Input: part model. Units: mm. Frame: model coordinates. A direction names the side the tool comes from. Coordinates: 2 decimals unless noted, no trailing zeros. Order: outer loops, then holes, each group sorted by start corner. A loop starts at its lowest first (then second) coordinate and runs counter-clockwise, first axis right, second up. Notation, with made-up numbers: (-25, 62.5) -> (-9, 62.5) arc R18 cw to (-9, 73.5) -> close; hole circle Ø2 at (49.5, 48). An arc over 180 degrees is marked (long way). One line per question, with ' | ' between items.
```python
from build123d import *

# Parameters (mm, degrees)
F1_DEPTH = 25.4
F3_DEPTH = 19.05


with BuildPart() as f1:
    # F0 (on Front) → F1 (new body)
    with BuildSketch(Plane.XZ):
        with BuildLine():
            Line((22.462801, 43.289483), (-25.703526, 43.289483))
            ThreePointArc((-25.703526, 43.289483), (-28.848755, 41.986686), (-30.151552, 38.841457))
            Line((-30.151552, 38.841457), (-30.151552, -42.523745))
            ThreePointArc((-30.151552, -42.523745), (-28.849641, -45.666835), (-25.706552, -46.968745))
            Line((-25.706552, -46.968745), (22.462801, -46.968745))
            ThreePointArc((22.462801, -46.968745), (25.605891, -45.666835), (26.907801, -42.523745))
            Line((26.907801, -42.523745), (26.907801, 38.844483))
            ThreePointArc((26.907801, 38.844483), (25.605891, 41.987572), (22.462801, 43.289483))
        make_face()
    extrude(amount=F1_DEPTH)

    # F2 (on face) → F3 (join)
    with BuildSketch(Plane.XZ.offset(25.4)):
        with BuildLine():
            Line((26.907801, 0), (-30.151552, 0))
            Line((-30.151552, 0), (-30.151552, -42.523745))
            ThreePointArc((-30.151552, -42.523745), (-28.849641, -45.666835), (-25.706552, -46.968745))
            Line((-25.706552, -46.968745), (22.462801, -46.968745))
            ThreePointArc((22.462801, -46.968745), (25.605891, -45.666835), (26.907801, -42.523745))
            Line((26.907801, -42.523745), (26.907801, 0))
        make_face()
    extrude(amount=F3_DEPTH)


solid = f1.part
```
1. Cut plane A-A, the plane y = -27.5. Return loops of the section in (x, z) (3 decimals), and give its area (3 significant figures).
Recorded:
outline: (-30.152, -42.524) arc R4.445 ccw to (-25.707, -46.969) -> (22.463, -46.969) arc R4.445 ccw to (26.908, -42.524) -> (26.908, 0) -> (-30.152, 0) -> close | area: 2,670 mm^2
2. Cut plane B-B, the plane x = 21.5. Return loops of the section in (y, z).
Recorded:
outline: (-44.45, -46.97) -> (0, -46.97) -> (0, 43.29) -> (-25.4, 43.29) -> (-25.4, 0) -> (-44.45, 0) -> close
3. Ray query, line 1 (Y direction, x = -21, z = 22); line 2 (Z direction, x = 13, y = -26.5); line 3 (Z direction, x = -27.5, y = -10). Return the intervals inside material, ascending. Write a range as [from, to].
Recorded:
line 1: y = [-25.4, 0] | line 2: z = [-46.97, 0] | line 3: z = [-46.59, 42.91]
4. Pin query (flat end, axial travel): pin 1 Ø5 at (x, y) = (18.5, -26) entering from +Z; pin 2 Ø9.5 at (x, y) = (6, -32) entering from +Z; pin 3 Ø21.5 at (x, z) = (10.5, 19.5) entering from -Y. Return the tip coordinate at first contact, or that it passes through.
Recorded:
pin 1: stops at z = 43.29 | pin 2: stops at z = 0 | pin 3: stops at y = -25.4
5. Cut plane C-C, the plane z = 31. Return loops of the section in (x, y), and give its area (3 significant figures).
Recorded:
outline: (-30.15, -25.4) -> (26.91, -25.4) -> (26.91, 0) -> (-30.15, 0) -> close | area: 1,450 mm^2
6. Access query for faces 1 (the face through (-2, -44.45, -23)), 2 (the face through (-2, -25.4, 22)). Directions: +Z, -Z, +X, -X, +Y, -Y. A direction counts if a zero-diameter tool reaches every point of the face in a straight line with its end or side. Return the directions, or none.
Recorded:
face 1: +Z, -Z, +X, -X, -Y | face 2: +Z, +X, -X, -Y
